Model file for the job. Use its own axes, mm. Face numbers are marked on the shaded views. A direction names the side the tool comes from. Give positions to 0.01 mm unless a question says otherwise; leave off trailing zeros. Loops run counter-clockwise (first coordinate to the right, second up) from the corner with the lowest first, then second, coordinate; pieces in that order, holes last. Notation, with made-up numbers: (27, -24.5) - (42, -24.5) arc R14 ccw to (42, -10.5) - close; hole circle Ø1 at (66, 44.25). An arc over 180 degrees is marked (long way). Answer as CSV lines item,"result". Start each with the question number.
Item 1: Drill centre lines: L1, parallel to X at y = -922, z = 0.15; L2, parallel to Y at x = -0.2, z = -2.6; L3, parallel to X at y = -916, z = 1.2. Where is each one in solid material? Low to high. Write a range as from..to.
Item 2: Saw through at B-B on z = 1.2. Give the cut face in (x, y).
Item 3: Saw through at A-A on x = 0. Give the cut face in (y, z).
Item 4: Tool access for the marked faces 1 and 2: list every direction of +Z, -Z, +X, -X, +Y, -Y with a clear straight run to the whole face (end or side of a thin tool).
Item 5: Saw through at C-C on y = -919.25. Give the cut face in (x, z), plus the area to 3 significant figures.
Item 6: Pin check, flat tips, straight feed: pin 1 (0.6 mm diameter, centred on x = -1, y = -920.5, fed in from +Z); pin 2 (1.5 mm diameter, centred on x = 0.5, y = -920.5, fed in from -Z); pin 3 (3 mm diameter, centred on x = -1, y = -915, fed in from +Z). Stop position of each tip, or through.
Item 7: Saw through at D-D on z = -0.75. Give the cut face in (x, y), plus the area to 3 significant figures.
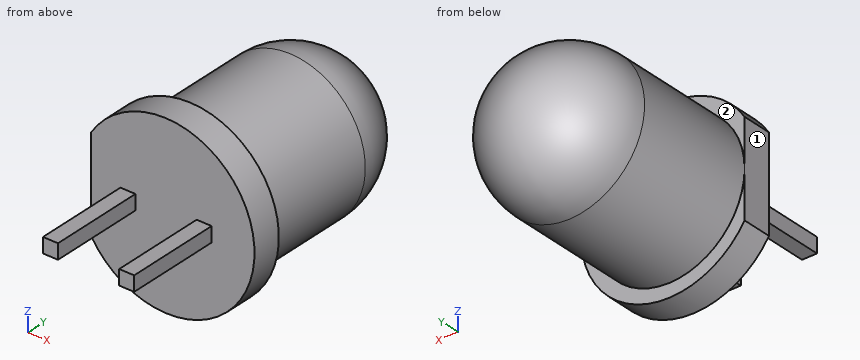
from build123d import *

# Parameters (mm, degrees)
CROQUIS3_W              = 0.5
CROQUIS3_H              = 0.5
SALIENTE_EXTRUIR3_DEPTH = 25.4
CROQUIS4_W              = 0.912534335
CROQUIS4_H              = 5.586103973
CORTAR_EXTRUIR1_DEPTH   = 25.4
CORTAR_EXTRUIR2_REACH   = 5.219
CROQUIS5_W              = 0.5
CROQUIS5_H              = 1
SKETCH1_W               = 3.04
SKETCH1_H               = 22.225
CUT_EXTRUDE1_DEPTH      = 4.181185999


with BuildPart() as part:
    # Croquis2 → Revolución1 (revolve)
    with BuildSketch(Plane(origin=(0, 0, 0), x_dir=(0, 0, -1), z_dir=(1, 0, 0))):
        with BuildLine():
            Line((0, -919.589259582), (2.95, -919.589259582))
            Line((2.95, -919.589259582), (2.95, -918.589259582))
            Line((2.95, -918.589259582), (2.5, -918.589259582))
            Line((2.5, -918.589259582), (2.5, -914.489259582))
            ThreePointArc((2.5, -914.489259582), (1.767766953, -912.721492629), (0, -911.989259582))
            Line((0, -911.989259582), (0, -919.589259582))
        make_face()
    revolve(axis=Axis((0, -1491.471633976, 0), (0, 1, 0)))

    # Croquis3 → Saliente-Extruir3 (add)
    with BuildSketch(Plane.XZ.offset(919.589259582)):
        with Locations((1.27, 0.018814001)):
            Rectangle(CROQUIS3_W, CROQUIS3_H)
        with Locations((-1.27, 0.018814001)):
            Rectangle(CROQUIS3_W, CROQUIS3_H)
    extrude(amount=SALIENTE_EXTRUIR3_DEPTH)

    # Croquis4 → Cortar-Extruir1 (cut)
    with BuildSketch(Plane(origin=(0, -918.589259582, 0), x_dir=(1, 0, 0), z_dir=(0, 1, 0))):
        with Locations((-2.956267168, 0.283432647)):
            Rectangle(CROQUIS4_W, CROQUIS4_H)
    extrude(amount=-CORTAR_EXTRUIR1_DEPTH, mode=Mode.SUBTRACT)

    # Croquis5 → Cortar-Extruir2 (cut, up to next)
    with BuildSketch(Plane.XY.offset(0.268814001), mode=Mode.PRIVATE) as cortar_extruir2_sk1:
        with Locations((-1.27, -944.489259582)):
            Rectangle(CROQUIS5_W, CROQUIS5_H)
    cortar_extruir2_tool1 = extrude(cortar_extruir2_sk1.sketch, amount=-CORTAR_EXTRUIR2_REACH, mode=Mode.PRIVATE) & part.part
    add(cortar_extruir2_tool1.solids().sort_by_distance((-1.27, -944.48926, 0.268814))[0], mode=Mode.SUBTRACT)

    # Sketch1 → Cut-Extrude1 (cut, through all)
    with BuildSketch(Plane(origin=(0, 0, -0.231185999), x_dir=(-1, 0, 0), z_dir=(0, 0, -1))):
        with Locations((0, -933.876759582)):
            Rectangle(SKETCH1_W, SKETCH1_H)
    extrude(amount=-CUT_EXTRUDE1_DEPTH, mode=Mode.SUBTRACT)


solid = part.part
Responses:
1,L1,"-1.52..-1.02, 1.02..1.52"
1,L2,"-919.59..-918.59"
1,L3,"-2.19..2.19"
2,outline,"(-2.5, -919.59) - (2.69, -919.59) - (2.69, -918.59) - (2.19, -918.59) - (2.19, -914.49) arc R2.19 ccw to (-2.19, -914.49) - (-2.19, -918.59) - (-2.5, -918.59) - close"
3,outline,"(-919.59, -2.95) - (-918.59, -2.95) - (-918.59, -2.5) - (-914.49, -2.5) arc R2.5 ccw to (-914.49, 2.5) - (-918.59, 2.5) - (-918.59, 2.95) - (-919.59, 2.95) - close"
4,face 1,"+Z, -Z, -X, +Y, -Y"
4,face 2,"+Y"
5,outline,"(-2.5, -1.57) arc R2.95 ccw (long way) to (-2.5, 1.57) - close"
5,area,"26.4 mm2"
6,pin 1,"z = 0.27"
6,pin 2,"z = -0.23"
6,pin 3,"z = 2.5"
7,outline,"(-2.5, -919.59) - (2.85, -919.59) - (2.85, -918.59) - (2.38, -918.59) - (2.38, -914.49) arc R2.38 ccw to (-2.38, -914.49) - (-2.38, -918.59) - (-2.5, -918.59) - close"
7,area,"33.8 mm2"
